Geometry check sheet. Reference: the model listing, model coordinates, mm. A direction names the side the tool comes from. Coordinates: 2 decimals unless noted, no trailing zeros. Loops run counter-clockwise (first coordinate to the right, second up) from the corner with the lowest first, then second, coordinate; pieces in that order, holes last.
from build123d import *

# Parameters (mm, degrees)
SKETCH_1_W          = 70
SKETCH_1_H          = 62
EXTRUDE_1_DEPTH     = 1
SKETCH_2_W          = 70
SKETCH_2_H          = 2
EXTRUDE_2_DEPTH     = 3.5
SKETCH_6_W          = 3
SKETCH_6_H          = 1
CUT_EXTRUDE_1_DEPTH = 71


with BuildPart() as part:
    # 草图1 → 凸台-拉伸1 (new body)
    with BuildSketch(Plane.XY):
        with Locations((-10.8, 14.6)):
            Rectangle(SKETCH_1_W, SKETCH_1_H)
    extrude(amount=EXTRUDE_1_DEPTH)

    # 草图2 → 凸台-拉伸2 (add)
    with BuildSketch(Plane.XY.offset(1)):
        with Locations((-10.8, 44.6)):
            Rectangle(SKETCH_2_W, SKETCH_2_H)
        with Locations((-10.8, -15.4)):
            Rectangle(SKETCH_2_W, SKETCH_2_H)
    extrude(amount=EXTRUDE_2_DEPTH)

    # 草图6 → 切除-拉伸1 (cut, through all)
    with BuildSketch(Plane.ZY.offset(45.8)):
        with Locations((2.5, 44.1)):
            Rectangle(SKETCH_6_W, SKETCH_6_H)
        with Locations((2.5, -14.9)):
            Rectangle(SKETCH_6_W, SKETCH_6_H)
    extrude(amount=-CUT_EXTRUDE_1_DEPTH, mode=Mode.SUBTRACT)


solid = part.part
1) Section check B-B on x = -28.5. Record the cut outline in (y, z), and give its area (3 significant figures).
Data:
outline: (-16.4, 0) - (45.6, 0) - (45.6, 4.5) - (43.6, 4.5) - (43.6, 4) - (44.6, 4) - (44.6, 1) - (-15.4, 1) - (-15.4, 4) - (-14.4, 4) - (-14.4, 4.5) - (-16.4, 4.5) - close
area: 70.0 mm2
2) Section check A-A on z = 2.75. Record the cut outline in (x, y).
Data:
outline: (-45.8, -16.4) - (24.2, -16.4) - (24.2, -15.4) - (-45.8, -15.4) - close; (-45.8, 44.6) - (24.2, 44.6) - (24.2, 45.6) - (-45.8, 45.6) - close
3) Mould release check, pull along Y, two halves, no side actions. Record for faces 1 (the flat face through (-11, -16.4, 2)), 2 (the flat face through (-11, 44.6, 2)), 3 (the flat face through (-11, 15, 0)): +Y half, -Y half, draft (parallel to the pull), parting line (faces both ways), or undercut.
Data:
face 1: -Y half
face 2: undercut
face 3: draft
4) Section check C-C on y = 13. Record the cut outline in (x, z), and give its area (3 significant figures).
Data:
outline: (-45.8, 0) - (24.2, 0) - (24.2, 1) - (-45.8, 1) - close
area: 70.0 mm2
5) Depth check by flat-ended pin: pin 1 (18 mm diameter, centred on x = -8.5, y = 21, fed in from +Z). Enter the tip coordinate at first touch or a pass-through.
Data:
pin 1: stops at z = 1
6) Access from +Z, -Z, +X, -X, +Y, -Y to the whole of each face (thin tool, end or side, straight path). Record for faces 4 (the flat face through (-11, -15.4, 2)), 5 (the flat face through (-11, -15, 4.5)).
Data:
face 4: +X, -X
face 5: +Z, +X, -X, +Y, -Y
7) Material ranges on probe 1 along Y at (x, z) = (9.5, 3.3); probe 2 along Z at (x, y) = (13.5, 8.5), recorded low to high.
Data:
probe 1: y = -16.4 to -15.4, 44.6 to 45.6
probe 2: z = 0 to 1
